Geometry: see drawing. Coordinates: mm, zero at the bounding-box minimum. Round coordinates to 2 decimals unless told otherwise and drop trailing zeros. Loops run counter-clockwise (first coordinate to the right, second up) from the corner with the lowest first, then second, coordinate; pieces in that order, holes last. Notation, with made-up numbers: (4, 73.25) - (35, 73.25) arc R16 cw to (35, 81.25) - close; hole circle Ø5 at (-29, 63.5). An arc over 180 degrees is marked (long way). Write item = value, one per line. Start each with the question number.
Item 1: Section A-A (x = 9.5). Return loops of the section in (y, z).
Item 2: Section D-D (z = 11). Return loops of the section in (x, y).
Item 3: Line query: line 1 (Z direction, x = 12, y = 8); line 2 (Y direction, x = 7.25, z = 5.5); line 3 (Y direction, x = 7.75, z = 1.5). Output: solid intervals per line, ascending. Write a range as from..to.
Item 4: Section C-C (y = 8.75). Return loops of the section in (x, z), plus the area to 3 significant figures.
Item 5: Draft query along Y for the marked faces 1 and 2. Return one class per face: pulls with the +Y half, pulls with the -Y half, needs draft (parallel to the pull), parting line crosses it, or undercut.
Item 6: First-contact query: pin 1 (5 mm diameter, centred on y = 8, z = 6, fed in from +X); pin 2 (1 mm diameter, centred on y = 4.5, z = 9, fed in from -X); pin 3 (2 mm diameter, centred on y = 9, z = 5.5, fed in from +X); pin 4 (5 mm diameter, centred on x = 14.5, z = 9.5, fed in from -Y). Flat tips, straight axial feed; report the tip coordinate or a pass-through.
Item 7: Section B-B (z = 5.75). Return loops of the section in (x, y), plus the area to 3 significant figures.
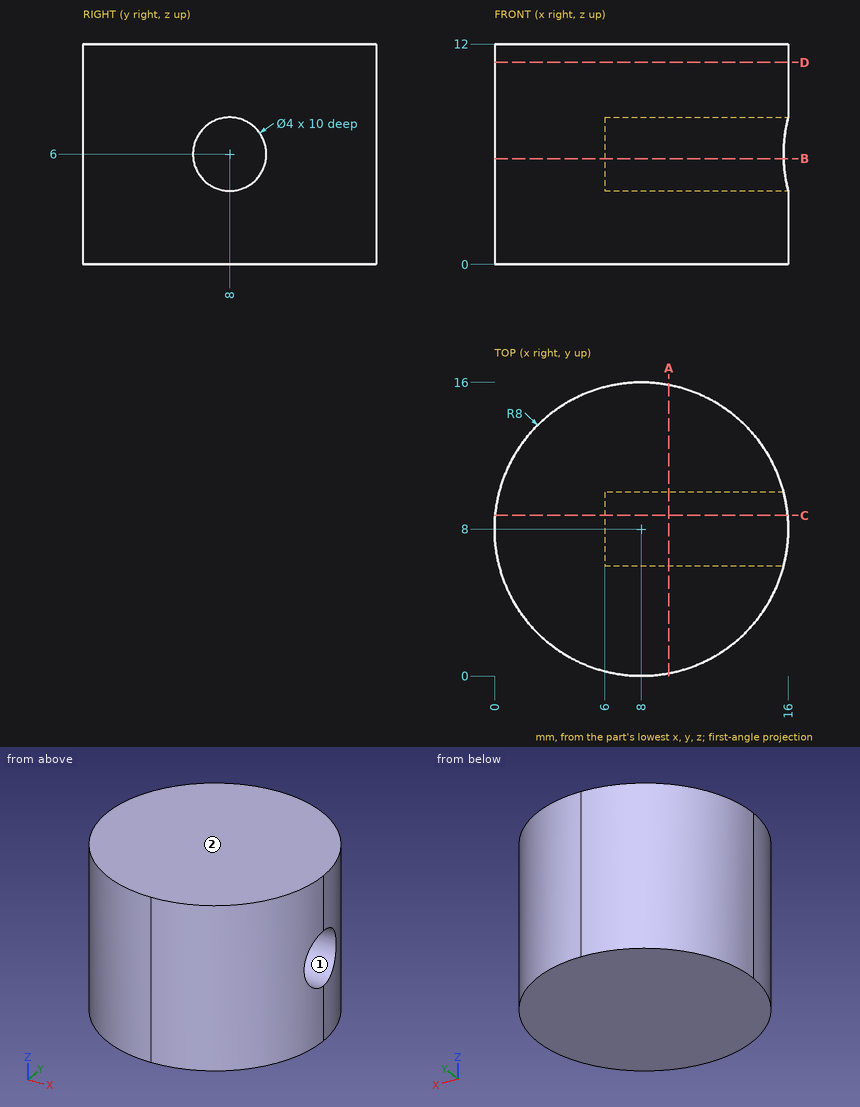
Taken from the geometry:
q1.outline = (0.14, 0) - (15.86, 0) - (15.86, 12) - (0.14, 12) - close; hole circle Ø4 at (8, 6)
q2.outline = circle Ø16 at (8, 8)
q3.line_1 = 0..4, 8..12
q3.line_2 = 0.04..6.06, 9.94..15.96
q3.line_3 = 0..16
q4.outline = (0.04, 0) - (15.96, 0) - (15.96, 4.15) - (6, 4.15) - (6, 7.85) - (15.96, 7.85) - (15.96, 12) - (0.04, 12) - close
q4.area = 154 mm^2
q5.face_1 = undercut
q5.face_2 = needs draft
q6.pin_1 = 16
q6.pin_2 = 0.58
q6.pin_3 = 15.87
q6.pin_4 = 1.07
q7.outline = (6, 6.02) - (6, 9.98) - (15.75, 9.98) arc R8 ccw (long way) to (15.75, 6.02) - close
q7.area = 162 mm^2
